Read the model definition and answer for the solid it produces. Units are mm, in the model's axes. A direction names the side the tool comes from. Round coordinates to 2 decimals unless told otherwise and drop trailing zeros. Write each loop counter-clockwise with the first axis right and the second up, starting at its lowest first coordinate (ties: lowest second). Pieces come first, ordered by that corner, then holes. Notation, with made-up numbers: (-32.75, 28.5) - (-26.75, 28.5) arc R31 ccw to (-26.75, 63.5) - close; hole circle Ø5 at (49, 62.25). An arc over 180 degrees is marked (long way). Use one line per item in the form item = value. Start each with the question number.
1) The part is cut by section B-B, the plane x = 0. Give the vertices of the cut face in (y, z).
2) Each of these flat-tipped pins is pushed along its axis until it touches: pin 1 (3 mm diameter, centred on x = 8, y = 2, fed in from +Z); pin 2 (5.5 mm diameter, centred on x = -2, y = -3, fed in from +Z); pin 3 (1.6 mm diameter, centred on y = 2.5, z = 3, fed in from -X). Where does it stop, or does it pass through?
3) The part is cut by section C-C, the plane y = -8.25. Give the vertices of the cut face in (x, z).
4) The part is cut by section D-D, the plane x = 7.75. Give the vertices of the cut face in (y, z).
5) For faces 1 (the face through (-0.1, -9, 4.5)), 2 (the face through (-7.719, 4.001, 4.715)), 3 (the face through (7.781, 3.876, 4.715)), determine the directions among +Z, -Z, +X, -X, +Y, -Y from which every point of the face is accessible in a straight line to the end or side of a thin tool.
6) The part is cut by section A-A, the plane y = 5. Give the vertices of the cut face in (x, z), plus the area to 3 significant figures.
7) For a pull along X with two mould halves and no side action, classify faces 4 (the face through (-5.5, 6.3, 4.5)), 5 (the face through (-5.5, -4.1, 4.5)), 6 (the face through (-8, 2, 2)), 7 (the face through (9.699, -9.715, 2.535)) as released by +X, released by -X, zero draft, split by the parting line, or undercut.
8) Consider line 1 along Y through (x, z) = (0, 2.05); line 2 along Y through (x, z) = (-3, 4.4); line 3 along X through (y, z) = (-5, 4.6). Determine where each line is inside the solid, lowest interval first. Write a range as from..to.
from build123d import *

# Parameters (mm, degrees)
SKETCH_1_W          = 20
SKETCH_1_H          = 20
EXTRUDE_1_DEPTH     = 5
SKETCH_2_W          = 11
SKETCH_2_H          = 18
SKETCH_2_R          = 1.25
CUT_EXTRUDE_1_DEPTH = 1
SKETCH_2_2_R        = 1.25
CUT_EXTRUDE_2_DEPTH = 6
SKETCH_3_W          = 4.5
SKETCH_3_H          = 2.7
SKETCH_3_H_2        = 2.574853583
CUT_EXTRUDE_3_DEPTH = 3
FILLET_1_R          = 1


with BuildPart() as part:
    # Эскиз1 → Бобышка-Вытянуть1 (new body)
    with BuildSketch(Plane.XY):
        Rectangle(SKETCH_1_W, SKETCH_1_H)
    extrude(amount=EXTRUDE_1_DEPTH)

    # Эскиз2 → Вырез-Вытянуть1 (cut)
    with BuildSketch(Plane.XY.offset(5)):
        Rectangle(SKETCH_2_W, SKETCH_2_H)
        with Locations((0, 5)):
            Circle(SKETCH_2_R, mode=Mode.SUBTRACT)
    extrude(amount=-CUT_EXTRUDE_1_DEPTH, mode=Mode.SUBTRACT)

    # Эскиз2<2> → Вырез-Вытянуть2 (cut, through all)
    with BuildSketch(Plane.XY.offset(5)):
        with Locations((0, 5)):
            Circle(SKETCH_2_2_R)
    extrude(amount=-CUT_EXTRUDE_2_DEPTH, mode=Mode.SUBTRACT)

    # Эскиз3 → Вырез-Вытянуть3 (cut)
    with BuildSketch(Plane.XY.offset(5)):
        with Locations((-7.75, 2.35)):
            Rectangle(SKETCH_3_W, SKETCH_3_H)
        with Locations((7.75, 2.287426792)):
            Rectangle(SKETCH_3_W, SKETCH_3_H_2)
    extrude(amount=-CUT_EXTRUDE_3_DEPTH, mode=Mode.SUBTRACT)

    # Скругление1
    fillet_1_edges = [part.edges().sort_by_distance(p)[0] for p in [
        (7.75, 1, 5),
        (7.75, 3.574853583, 5),
        (-7.75, 1, 5),
        (-7.75, 3.7, 5),
        (-10, -10, 2.5),
        (10, -10, 2.5),
        (10, 10, 2.5),
        (-10, 10, 2.5),
    ]]
    fillet(fillet_1_edges, radius=FILLET_1_R)


solid = part.part
Geometry results:
q1.outline = (-10, 0) - (3.75, 0) - (3.75, 4) - (-9, 4) - (-9, 5) - (-10, 5) - close; (6.25, 0) - (10, 0) - (10, 5) - (9, 5) - (9, 4) - (6.25, 4) - close
q2.pin_1 = 4.87
q2.pin_2 = 4
q2.pin_3 = -5.5
q3.outline = (-10, 0) - (10, 0) - (10, 5) - (5.5, 5) - (5.5, 4) - (-5.5, 4) - (-5.5, 5) - (-10, 5) - close
q4.outline = (-10, 0) - (10, 0) - (10, 5) - (4.57, 5) arc R1 ccw to (3.57, 4) - (3.57, 2) - (1, 2) - (1, 4) arc R1 ccw to (0, 5) - (-10, 5) - close
q5.face_1 = +Z
q5.face_2 = +Z, -X
q5.face_3 = +Z, +X, -X
q6.outline = (-10, 0) - (-1.25, 0) - (-1.25, 4) - (-5.5, 4) - (-5.5, 5) - (-10, 5) - close; (1.25, 0) - (10, 0) - (10, 5) - (5.5, 5) - (5.5, 4) - (1.25, 4) - close
q6.area = 79.0 mm2
q7.face_4 = undercut
q7.face_5 = undercut
q7.face_6 = zero draft
q7.face_7 = released by +X
q8.line_1 = -10..3.75, 6.25..10
q8.line_2 = -10..-9, 9..10
q8.line_3 = -10..-5.5, 5.5..10
